from build123d import *

# Parameters (mm, degrees)
SKETCH3_W                    = 114
SKETCH3_H                    = 40
BASE_FLANGE1_DEPTH           = 3
EDGE_FLANGE1_STRIP_W         = 13.4732
EDGE_FLANGE1_STRIP_H         = 3
EDGE_FLANGE1_STRIP_CUT_DEPTH = 40
EDGE_FLANGE1_DEPTH           = 40
EDGE_FLANGE2_STRIP_W         = 13.4732
EDGE_FLANGE2_STRIP_H         = 3
EDGE_FLANGE2_STRIP_CUT_DEPTH = 40
EDGE_FLANGE2_DEPTH           = 40
SKETCH11_R                   = 8
SKETCH11_R_2                 = 2
CUT_EXTRUDE1_DEPTH           = 10
CUT_EXTRUDE2_REACH           = 157.592
SKETCH12_R                   = 2
CUT_EXTRUDE3_DEPTH           = 156.592416268
CUT_EXTRUDE3_DEPTH_BACK      = 156.592416268
CUT_EXTRUDE4_DEPTH           = 10
FILLET1_R                    = 1


# Sheet-metal steps are written as plain solids
with BuildPart() as part:
    # Sketch3 → Base-Flange1 (new body)
    with BuildSketch(Plane(origin=(0, 0, 0), x_dir=(1, 0, 0), z_dir=(0, 1, 0))):
        Rectangle(SKETCH3_W, SKETCH3_H)
    extrude(amount=-BASE_FLANGE1_DEPTH)

    # Edge-Flange1 strip (across the edge) → Edge-Flange1 strip cut (cut)
    with BuildSketch(Plane(origin=(-57, 0, -20), x_dir=(1, 0, 0), z_dir=(0, 0, 1))):
        with Locations((-6, -1.5)):
            Rectangle(EDGE_FLANGE1_STRIP_W, EDGE_FLANGE1_STRIP_H)
    extrude(amount=EDGE_FLANGE1_STRIP_CUT_DEPTH, mode=Mode.SUBTRACT)

    # Edge-Flange1 section (across the edge) → Edge-Flange1 (add)
    with BuildSketch(Plane(origin=(-57, 0, -20), x_dir=(1, 0, 0), z_dir=(0, 0, 1))):
        with BuildLine():
            Line((-3, 0.7366), (-3, 97))
            Line((-3, 97), (0, 97))
            Line((0, 97), (0, 0.7366))
            ThreePointArc((0, 0.7366), (0.215745145, 0.215745145), (0.7366, 0))
            Line((0.7366, 0), (0.7366, -3))
            ThreePointArc((0.7366, -3), (-1.905575199, -1.905575199), (-3, 0.7366))
        make_face()
    extrude(amount=EDGE_FLANGE1_DEPTH)

    # Edge-Flange2 strip (across the edge) → Edge-Flange2 strip cut (cut)
    with BuildSketch(Plane(origin=(57, 0, 20), x_dir=(-1, 0, 0), z_dir=(0, 0, -1))):
        with Locations((-6, -1.5)):
            Rectangle(EDGE_FLANGE2_STRIP_W, EDGE_FLANGE2_STRIP_H)
    extrude(amount=EDGE_FLANGE2_STRIP_CUT_DEPTH, mode=Mode.SUBTRACT)

    # Edge-Flange2 section (across the edge) → Edge-Flange2 (add)
    with BuildSketch(Plane(origin=(57, 0, 20), x_dir=(-1, 0, 0), z_dir=(0, 0, -1))):
        with BuildLine():
            Line((-3, 0.7366), (-3, 97))
            Line((-3, 97), (0, 97))
            Line((0, 97), (0, 0.7366))
            ThreePointArc((0, 0.7366), (0.215745145, 0.215745145), (0.7366, 0))
            Line((0.7366, 0), (0.7366, -3))
            ThreePointArc((0.7366, -3), (-1.905575199, -1.905575199), (-3, 0.7366))
        make_face()
    extrude(amount=EDGE_FLANGE2_DEPTH)

    # Sketch11 → Cut-Extrude1 (cut)
    with BuildSketch(Plane(origin=(0, -3, 0), x_dir=(-1, 0, 0), z_dir=(0, -1, 0))):
        with Locations(Location((0, 0, 0), (0, 0, 90))):
            Circle(SKETCH11_R)
        with Locations(Location((12.727922061, 12.727922061, 0), (0, 0, 90))):
            Circle(SKETCH11_R_2)
        with Locations(Location((12.727922061, -12.727922061, 0), (0, 0, 90))):
            Circle(SKETCH11_R_2)
        with Locations(Location((-12.727922061, -12.727922061, 0), (0, 0, 90))):
            Circle(SKETCH11_R_2)
        with Locations(Location((-12.727922061, 12.727922061, 0), (0, 0, 90))):
            Circle(SKETCH11_R_2)
        with Locations(Location((50.2634, 6.666666667, 0), (0, 0, 90))):
            Circle(SKETCH11_R_2)
        with Locations(Location((-50.2634, 6.666666667, 0), (0, 0, 90))):
            Circle(SKETCH11_R_2)
        with Locations(Location((50.2634, -6.666666667, 0), (0, 0, 90))):
            Circle(SKETCH11_R_2)
        with Locations(Location((-50.2634, -6.666666667, 0), (0, 0, 90))):
            Circle(SKETCH11_R_2)
    extrude(amount=-CUT_EXTRUDE1_DEPTH, mode=Mode.SUBTRACT)

    # Cut-Extrude2: up to this face of the body (flat: up to its plane)
    cut_extrude2_end = Plane(part.part.faces().sort_by_distance((-60, 48.8683, 0))[0])
    # Sketch12 → Cut-Extrude2 (cut, up to the picked face)
    with BuildSketch(Plane(origin=(60, 0, 0), x_dir=(0, 0, -1), z_dir=(1, 0, 0)), mode=Mode.PRIVATE) as cut_extrude2_sk1:
        with Locations(Location((12.5, 79.674243403, 0), (0, 0, 90))):
            Circle(SKETCH12_R)
    cut_extrude2_tool1 = split(extrude(cut_extrude2_sk1.sketch, amount=-CUT_EXTRUDE2_REACH, mode=Mode.PRIVATE), bisect_by=cut_extrude2_end, keep=Keep.BOTH, mode=Mode.PRIVATE)
    # Sketch12 → Cut-Extrude2 (cut, up to the picked face)
    with BuildSketch(Plane(origin=(60, 0, 0), x_dir=(0, 0, -1), z_dir=(1, 0, 0)), mode=Mode.PRIVATE) as cut_extrude2_sk2:
        with Locations(Location((12.5, 90.674243403, 0), (0, 0, 90))):
            Circle(SKETCH12_R)
    cut_extrude2_tool2 = split(extrude(cut_extrude2_sk2.sketch, amount=-CUT_EXTRUDE2_REACH, mode=Mode.PRIVATE), bisect_by=cut_extrude2_end, keep=Keep.BOTH, mode=Mode.PRIVATE)
    # Sketch12 → Cut-Extrude2 (cut, up to the picked face)
    with BuildSketch(Plane(origin=(60, 0, 0), x_dir=(0, 0, -1), z_dir=(1, 0, 0)), mode=Mode.PRIVATE) as cut_extrude2_sk3:
        with Locations(Location((-12.5, 79.674243403, 0), (0, 0, 90))):
            Circle(SKETCH12_R)
    cut_extrude2_tool3 = split(extrude(cut_extrude2_sk3.sketch, amount=-CUT_EXTRUDE2_REACH, mode=Mode.PRIVATE), bisect_by=cut_extrude2_end, keep=Keep.BOTH, mode=Mode.PRIVATE)
    # Sketch12 → Cut-Extrude2 (cut, up to the picked face)
    with BuildSketch(Plane(origin=(60, 0, 0), x_dir=(0, 0, -1), z_dir=(1, 0, 0)), mode=Mode.PRIVATE) as cut_extrude2_sk4:
        with Locations(Location((-12.5, 90.674243403, 0), (0, 0, 90))):
            Circle(SKETCH12_R)
    cut_extrude2_tool4 = split(extrude(cut_extrude2_sk4.sketch, amount=-CUT_EXTRUDE2_REACH, mode=Mode.PRIVATE), bisect_by=cut_extrude2_end, keep=Keep.BOTH, mode=Mode.PRIVATE)
    add(cut_extrude2_tool1.solids().sort_by(Axis((60, 79.674243, -12.5), (-1, 0, 0)))[0], mode=Mode.SUBTRACT)
    add(cut_extrude2_tool2.solids().sort_by(Axis((60, 90.674243, -12.5), (-1, 0, 0)))[0], mode=Mode.SUBTRACT)
    add(cut_extrude2_tool3.solids().sort_by(Axis((60, 79.674243, 12.5), (-1, 0, 0)))[0], mode=Mode.SUBTRACT)
    add(cut_extrude2_tool4.solids().sort_by(Axis((60, 90.674243, 12.5), (-1, 0, 0)))[0], mode=Mode.SUBTRACT)

    # Sketch14 → Cut-Extrude3 (cut, two sides: drawn at the far end of the back side and taken through both)
    with BuildSketch(Plane(origin=(60, 0, 0), x_dir=(0, 0, -1), z_dir=(1, 0, 0)).offset(-CUT_EXTRUDE3_DEPTH_BACK)):
        Polygon((-12.5, 60.805943605), (-1.641411821, 36.3683), (-12.5, 11.930656395), align=None)
        Polygon((-10.858588179, 64.5), (0, 40.062356395), (10.858588179, 64.5), align=None)
        Polygon((12.5, 60.805943605), (1.641411821, 36.3683), (12.5, 11.930656395), align=None)
        Polygon((10.858588179, 8.2366), (0, 32.674243605), (-10.858588179, 8.2366), align=None)
    extrude(amount=CUT_EXTRUDE3_DEPTH + CUT_EXTRUDE3_DEPTH_BACK, mode=Mode.SUBTRACT)

    # Sketch15 → Cut-Extrude4 (cut)
    with BuildSketch(Plane.XZ.offset(3)):
        Polygon((19.727922061, 12.878679656), (32.606601718, 0), (19.727922061, -12.878679656), align=None)
        Polygon((21.849242405, 15), (34.727922061, 2.121320344), (47.606601718, 15), align=None)
        Polygon((44.2634, 7.414157595), (36.849242405, 0), (44.2634, -7.414157595), align=None)
        Polygon((47.606601718, -15), (34.727922061, -2.121320344), (21.849242405, -15), align=None)
        Polygon((-21.849242405, -15), (-47.606601718, -15), (-34.727922061, -2.121320344), align=None)
        Polygon((-44.2634, -7.414157595), (-44.2634, 7.414157595), (-36.849242405, 0), align=None)
        Polygon((-47.606601718, 15), (-21.849242405, 15), (-34.727922061, 2.121320344), align=None)
        Polygon((-19.727922061, -12.878679656), (-19.727922061, 12.878679656), (-32.606601718, 0), align=None)
    extrude(amount=-CUT_EXTRUDE4_DEPTH, mode=Mode.SUBTRACT)

    # Fillet1
    fillet1_edges = [part.edges().sort_by_distance(p)[0] for p in [
        (58.5, 60.805943605, -12.5),
        (-58.5, 60.805943605, -12.5),
        (58.5, 11.930656395, -12.5),
        (-58.5, 11.930656395, -12.5),
        (58.5, 36.3683, -1.641411821),
        (-58.5, 36.3683, -1.641411821),
        (58.5, 64.5, 10.858588179),
        (-58.5, 64.5, 10.858588179),
        (58.5, 64.5, -10.858588179),
        (-58.5, 64.5, -10.858588179),
        (58.5, 40.062356395, 0),
        (-58.5, 40.062356395, 0),
        (58.5, 8.2366, -10.858588179),
        (-58.5, 8.2366, -10.858588179),
        (58.5, 8.2366, 10.858588179),
        (-58.5, 8.2366, 10.858588179),
        (58.5, 32.674243605, 0),
        (-58.5, 32.674243605, 0),
        (58.5, 11.930656395, 12.5),
        (-58.5, 11.930656395, 12.5),
        (58.5, 60.805943605, 12.5),
        (-58.5, 60.805943605, 12.5),
        (58.5, 36.3683, 1.641411821),
        (-58.5, 36.3683, 1.641411821),
        (-34.727922061, -1.5, -2.121320344),
        (-21.849242405, -1.5, -15),
        (-47.606601718, -1.5, -15),
        (47.606601718, -1.5, -15),
        (21.849242405, -1.5, -15),
        (34.727922061, -1.5, -2.121320344),
        (21.849242405, -1.5, 15),
        (47.606601718, -1.5, 15),
        (34.727922061, -1.5, 2.121320344),
        (44.2634, -1.5, 7.414157595),
        (44.2634, -1.5, -7.414157595),
        (36.849242405, -1.5, 0),
        (-19.727922061, -1.5, -12.878679656),
        (-32.606601718, -1.5, 0),
        (-19.727922061, -1.5, 12.878679656),
        (-36.849242405, -1.5, 0),
        (-44.2634, -1.5, -7.414157595),
        (-44.2634, -1.5, 7.414157595),
        (-34.727922061, -1.5, 2.121320344),
        (-47.606601718, -1.5, 15),
        (-21.849242405, -1.5, 15),
        (19.727922061, -1.5, -12.878679656),
        (19.727922061, -1.5, 12.878679656),
        (32.606601718, -1.5, 0),
    ]]
    fillet(fillet1_edges, radius=FILLET1_R)


solid = part.part
Here's how the part is built. I have some questions about the finished solid (model axes, mm). A direction names the side the tool comes from. Round coordinates to 2 decimals unless told otherwise and drop trailing zeros. Order: outer loops, then holes, each group sorted by start corner. A loop starts at its lowest first (then second) coordinate and runs counter-clockwise, first axis right, second up. Notation, with made-up numbers: M 79.25,-30.5 L 94.25,-30.5 A30 cw 94.25,0.5 Z; hole C -2,71 d4. An arc over 180 degrees is marked long. One line per question, with ' | ' between items.
1) Imagine slicing it at B-B, the plane y = 20.5. Count the separate pieces of the cut face and the enclosed holes in it, plus the area to 3 significant figures.
Checked values:
separate pieces: 8 | enclosed holes: 0 | area: 129 mm²
2) Imagine slicing it at C-C, the plane x = 41. Write out the boundary of the cut face in (y, z), plus the area to 3 significant figures.
Checked values:
outline: M -3,-20 L 0,-20 L 0,-15 L -3,-15 Z; M -3,-8.39 L 0,-8.39 L 0,-4.15 L -3,-4.15 Z; M -3,4.15 L 0,4.15 L 0,8.39 L -3,8.39 Z; M -3,15 L 0,15 L 0,20 L -3,20 Z | area: 55.5 mm²
3) I need wall thicknesses on line 1 (X direction, y = 46, z = 13); line 2 (Y direction, x = -58, z = -12); line 3 (Y direction, x = 42.5, z = 9). Which ranges of each line are inside material? Lowest first, please.
Checked values:
line 1: x = -60 to -57, 57 to 60 | line 2: y = -2.57 to 15.78, 56.96 to 77.74, 81.61 to 88.74, 92.61 to 97 | line 3: y = -3 to 0
4) On a 3-axis mill with a long thin cutter (end or side, diameter ignored), from which of +Z, -Z, +X, -X, +Y, -Y can I reach the whole of each face in a straight line? I mean faces 1 (the flat face through (58.479, 46.775, 6.265)), 2 (the flat face through (-35, -2, 15)), 3 (the flat face through (-57, 50, -5)). Say none if no direction works.
Checked values:
face 1: +X, -X | face 2: +Y, -Y | face 3: +Z, -Z, +Y
5) Imagine slicing it at A-A, the plane x = 0. Write out the boundary of the cut face in (y, z).
Checked values:
outline: M -3,-20 L 0,-20 L 0,-8 L -3,-8 Z; M -3,8 L 0,8 L 0,20 L -3,20 Z
6) I'm going to push flat-ended pins straight in: pin 1 Ø0.9 at (x, z) = (58, 3.5) entering from -Y; pin 2 Ø3.5 at (y, z) = (79.67, -12.5) entering from +X; pin 3 Ø1.5 at (x, z) = (-58, -1.5) entering from -Y; pin 4 Ø2.5 at (y, z) = (-1.5, -2) entering from +X. Where does each tip first touch, or does it pass through?
Checked values:
pin 1: stops at y = -2.77 | pin 2: passes through | pin 3: stops at y = -2.87 | pin 4: stops at x = 59.87
7) We'd pull the mould along X, two halves only. Please class faces 4 (the cylindrical face through (-58.88, -1.93, -0.28)), 5 (the cylindrical face through (58.88, -1.93, 0.28)), 6 (the flat face through (-40.02, -1.52, -3.17)), 7 (the flat face through (-59, 36, -12.5)): released by +X, released by -X, zero draft, split by the parting line, or undercut.
Checked values:
face 4: released by -X | face 5: released by +X | face 6: undercut | face 7: zero draft
